Check sheet for the drawn part. Datum: minimum x, y, z corner. Units: mm. A direction names the side the tool comes from. Give positions to 0.01 mm unless a question says otherwise; leave off trailing zeros. Order: outer loops, then holes, each group sorted by start corner. A loop starts at its lowest first (then second) coordinate and runs counter-clockwise, first axis right, second up.
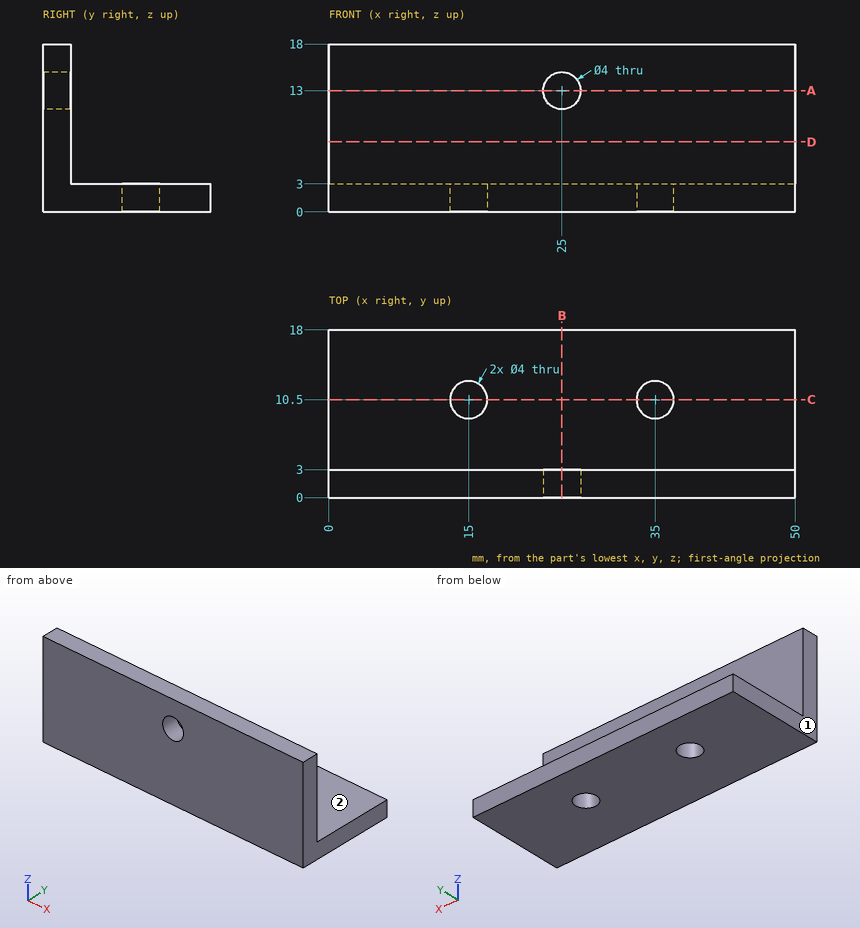
Item 1: Scan lines: L1, parallel to X at y = 1.95, z = 13; L2, parallel to Y at x = 15, z = 1.95; L3, parallel to Y at x = 14, z = 5.5. Record each from-to range of solid material in increasing order.
Reported:
L1: x = 0 to 23, 27 to 50
L2: y = 0 to 8.5, 12.5 to 18
L3: y = 0 to 3
Item 2: Sectioned sample at B-B (x = 25). Enter the section's corners in (y, z).
Reported:
outline: (0, 0) - (18, 0) - (18, 3) - (3, 3) - (3, 11) - (0, 11) - close; (0, 15) - (3, 15) - (3, 18) - (0, 18) - close
Item 3: Sectioned sample at D-D (z = 7.5). Enter the section's corners in (x, y), and give its area (3 significant figures).
Reported:
outline: (0, 0) - (50, 0) - (50, 3) - (0, 3) - close
area: 150 mm2
Item 4: Sectioned sample at A-A (z = 13). Enter the section's corners in (x, y).
Reported:
outline: (0, 0) - (23, 0) - (23, 3) - (0, 3) - close; (27, 0) - (50, 0) - (50, 3) - (27, 3) - close
Item 5: Gauge pin test, flat ends, axial feed: pin 1 (2.5 mm diameter, centred on x = 25, z = 13, fed in from -Y); pin 2 (5 mm diameter, centred on x = 20, y = 13, fed in from +Z); pin 3 (2 mm diameter, centred on x = 28.5, z = 7, fed in from +Y). Record the tip position at first contact, or that the pin passes through.
Reported:
pin 1: passes through
pin 2: stops at z = 3
pin 3: stops at y = 3
Item 6: Set-up check for the marked faces 1 and 2: record each of +Z, -Z, +X, -X, +Y, -Y from which the full face is reachable in a straight line by a thin tool's end or side.
Reported:
face 1: +Z, -Z, -X, +Y, -Y
face 2: +Z, +X, -X, +Y
Item 7: Sectioned sample at C-C (y = 10.5). Enter the section's corners in (x, z), and give its area (3 significant figures).
Reported:
outline: (0, 0) - (13, 0) - (13, 3) - (0, 3) - close; (17, 0) - (33, 0) - (33, 3) - (17, 3) - close; (37, 0) - (50, 0) - (50, 3) - (37, 3) - close
area: 126 mm2
